Verification items for the finished model (mm, model axes). Face numbers are marked on the shaded views. A direction names the side the tool comes from. Coordinates: 2 decimals unless noted, no trailing zeros. Loops run counter-clockwise (first coordinate to the right, second up) from the corner with the lowest first, then second, coordinate; pieces in that order, holes last. Notation, with made-up numbers: (-37.5, 54) - (13.5, 54) arc R16 cw to (13.5, 84) - close; hole circle Ø7 at (-9.5, -28). An arc over 180 degrees is marked (long way). Answer as CSV lines item,"result". Start each with the question number.
1. Cross-section at A-A (x = 0). Enter the section's corners in (y, z), plus the area to 3 significant figures.
2. Gauge pin test, flat ends, axial feed: P1, Ø1.2, axis at x = -1, z = 5.5, coming from the -Y side; P2, Ø3.5, axis at x = 1.5, y = 0, coming from the +Z side; P3, Ø4, axis at y = -3, z = 1, coming from the -X side. Record the tip position at first contact, or that the pin passes through.
3. Material ranges on line 1 (Z direction, x = 3.5, y = -4); line 2 (Z direction, x = 2, y = -2.25); line 3 (X direction, y = 2, z = -23.5), recorded low to high. Write a range as [from, to].
4. Cross-section at B-B (z = -5). Enter the section's corners in (x, y), plus the area to 3 significant figures.
5. Release check for a two-part mould opening along X. For the marked faces 1, 2 and 3 record: pulls with the +X half, pulls with the -X half, needs draft (parallel to the pull), parting line crosses it, or undercut.
6. Set-up check for the marked faces 4, 5 and 6: record each of +Z, -Z, +X, -X, +Y, -Y from which the full face is reachable in a straight line by a thin tool's end or side.
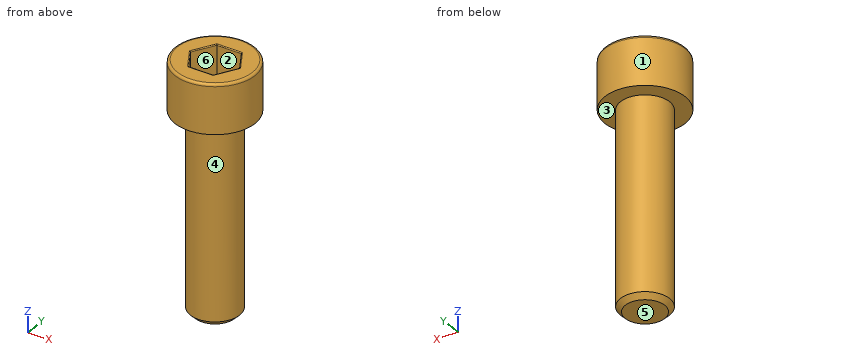
```python
from build123d import *

# Parameters (mm, degrees)
ESQUISSE1_R             = 6.5
BASE_EXTRUSION_DEPTH    = 8
ENL_V_MAT_EXTRU_1_DEPTH = 5
CONG_1_R                = 0.4
CONG_2_R                = 0.15
ESQUISSE3_R             = 4
BOSS_EXTRU_1_DEPTH      = 32
CHANFREIN1_SIZE         = 0.8


with BuildPart() as part:
    # Esquisse1 → Base-Extrusion (new body)
    with BuildSketch(Plane.XY):
        Circle(ESQUISSE1_R)
    extrude(amount=BASE_EXTRUSION_DEPTH)

    # Esquisse2 → Enlèv. mat.-Extru.1 (cut)
    with BuildSketch(Plane.XY.offset(8)):
        Polygon((-4, 0), (-2.004145082, 3.461705142), (2.004145082, 3.461705142), (4, 0), (2.004145082, -3.461705142), (-2.004145082, -3.461705142), align=None)
    extrude(amount=-ENL_V_MAT_EXTRU_1_DEPTH, mode=Mode.SUBTRACT)

    # Congé1
    cong_1_edges = [part.edges().sort_by_distance(p)[0] for p in [
        (-6.5, 0, 8),
    ]]
    fillet(cong_1_edges, radius=CONG_1_R)

    # Congé2
    cong_2_edges = [part.edges().sort_by_distance(p)[0] for p in [
        (-3.002072541, -1.730852571, 8),
        (0, -3.461705142, 8),
        (3.002072541, -1.730852571, 8),
        (3.002072541, 1.730852571, 8),
        (0, 3.461705142, 8),
        (-3.002072541, 1.730852571, 8),
    ]]
    fillet(cong_2_edges, radius=CONG_2_R)

    # Esquisse3 → Boss.-Extru.1 (add)
    with BuildSketch(Plane(origin=(0, 0, 0), x_dir=(-1, 0, 0), z_dir=(0, 0, -1))):
        Circle(ESQUISSE3_R)
    extrude(amount=BOSS_EXTRU_1_DEPTH)

    # Chanfrein1
    chanfrein1_edges = [part.edges().sort_by_distance(p)[0] for p in [
        (4, 0, -32),
    ]]
    chamfer(chanfrein1_edges, length=CHANFREIN1_SIZE)


solid = part.part
```
Values follow:
1,outline,"(-6.5, 0) - (-4, 0) - (-4, -31.2) - (-3.2, -32) - (3.2, -32) - (4, -31.2) - (4, 0) - (6.5, 0) - (6.5, 7.6) arc R0.4 ccw to (6.1, 8) - (3.61, 8) arc R0.15 ccw to (3.46, 7.85) - (3.46, 3) - (-3.46, 3) - (-3.46, 7.85) arc R0.15 ccw to (-3.61, 8) - (-6.1, 8) arc R0.4 ccw to (-6.5, 7.6) - close"
1,area,"325 mm²"
2,P1,"stops at y = -6.49"
2,P2,"stops at z = 3"
2,P3,"stops at x = -6.42"
3,line 1,"z = [0, 8]"
3,line 2,"z = [-32, 3]"
3,line 3,"x = [-3.46, 3.46]"
4,outline,"circle Ø8 at (0, 0)"
4,area,"50.3 mm²"
5,face 1,"parting line crosses it"
5,face 2,"undercut"
5,face 3,"needs draft"
6,face 4,"-Z"
6,face 5,"-Z, +X, -X, +Y, -Y"
6,face 6,"+Z"
